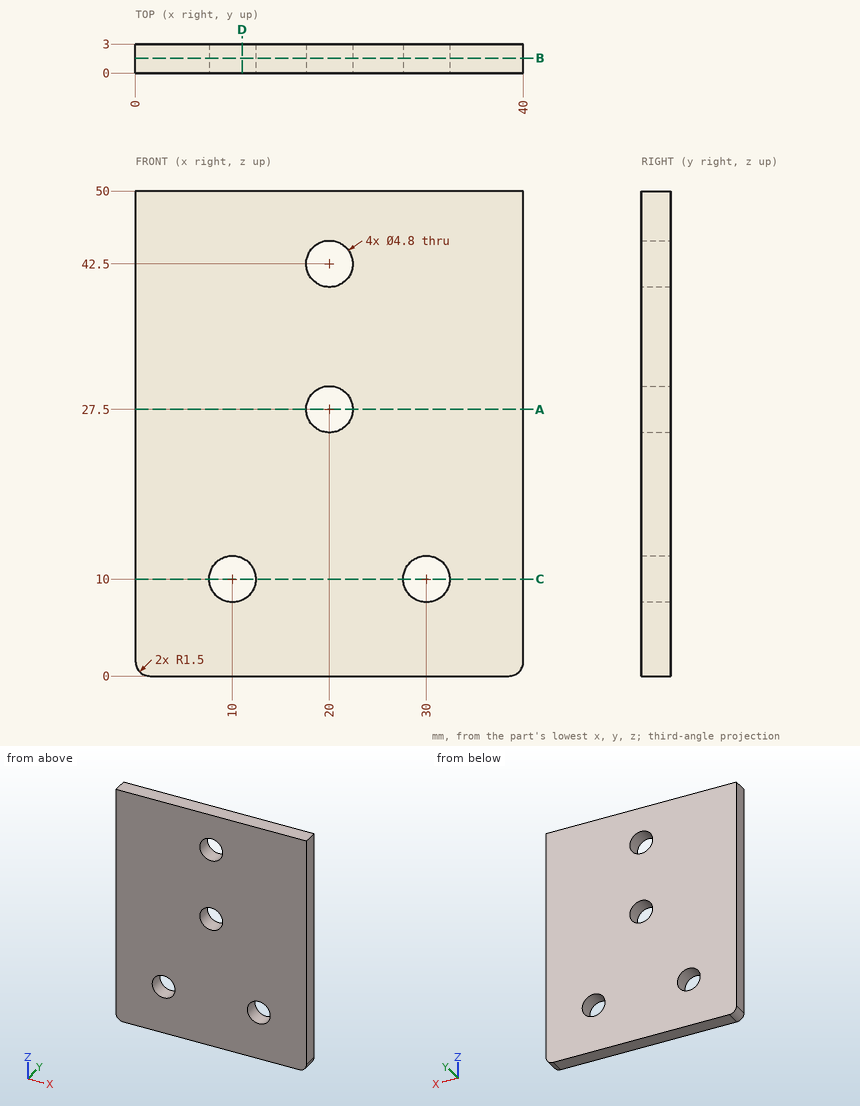
Geometry check sheet. Reference: drawing and pictorial views, mm from the part's lowest x, y, z. Round coordinates to 2 decimals unless told otherwise and drop trailing zeros. Order: outer loops, then holes, each group sorted by start corner. A loop starts at its lowest first (then second) coordinate and runs counter-clockwise, first axis right, second up. Notation, with made-up numbers: M 7,29.25 L 48,29.25 A10 ccw 48,40.25 Z; hole C 74,-0.75 d8. An arc over 180 degrees is marked long. Answer in a Markdown table with one row per item.
(1) Scan lines: probe 1 along X at (y, z) = (2.45, 10); probe 2 along Z at (x, y) = (18.5, 1.8); probe 3 along X at (y, z) = (2.05, 42.5). Record each from-to range of solid material in increasing order. Write a range as from..to.
Responses:
| item | result |
|---|---|
| probe 1 | x = 0..7.6, 12.4..27.6, 32.4..40 |
| probe 2 | z = 0..25.63, 29.37..40.63, 44.37..50 |
| probe 3 | x = 0..17.6, 22.4..40 |
(2) Sectioned sample at C-C, the plane z = 10. Record the cut outline in (x, y), and give its area (3 significant figures).
Responses:
| item | result |
|---|---|
| outline | M 0,0 L 7.6,0 L 7.6,3 L 0,3 Z; M 12.4,0 L 27.6,0 L 27.6,3 L 12.4,3 Z; M 32.4,0 L 40,0 L 40,3 L 32.4,3 Z |
| area | 91.2 mm² |
(3) Sectioned sample at A-A, the plane z = 27.5. Record the cut outline in (x, y), and give its area (3 significant figures).
Responses:
| item | result |
|---|---|
| outline | M 0,0 L 17.6,0 L 17.6,3 L 0,3 Z; M 22.4,0 L 40,0 L 40,3 L 22.4,3 Z |
| area | 106 mm² |
(4) Sectioned sample at D-D, the plane x = 11. Record the cut outline in (y, z).
Responses:
| item | result |
|---|---|
| outline | M 0,0 L 3,0 L 3,7.82 L 0,7.82 Z; M 0,12.18 L 3,12.18 L 3,50 L 0,50 Z |
(5) Sectioned sample at B-B, the plane y = 1.55. Record the cut outline in (x, z).
Responses:
| item | result |
|---|---|
| outline | M 0,1.5 A1.5 ccw 1.5,0 L 38.5,0 A1.5 ccw 40,1.5 L 40,50 L 0,50 Z; hole C 10,10 d4.8; hole C 20,27.5 d4.8; hole C 20,42.5 d4.8; hole C 30,10 d4.8 |
